Read the model definition and answer for the solid it produces. Units are mm, in the model's axes. A direction names the side the tool comes from. Round coordinates to 2 decimals unless told otherwise and drop trailing zeros. Order: outer loops, then holes, each group sorted by start corner. A loop starts at its lowest first (then second) coordinate and runs counter-clockwise, first axis right, second up. Notation, with made-up numbers: (30.5, 15) - (61.5, 15) arc R17 ccw to (61.5, 29) - close; hole circle Ø7 at (67, 80.25). An arc over 180 degrees is marked (long way). Answer as a JSON object with one key per item and string values. Group by question number.
Q1. Given pin 1 Ø5 at (x, y) = (292.43, 215.24) entering from -Z, flat-ended and moving along its own axis, determine where the tip first touches the part or whether it passes through.
Q2. Consider line 1 (Y direction, x = 303, z = 1.35); line 2 (Y direction, x = 310.5, z = 2.5); line 3 (Y direction, x = 301, z = 1.7). Determine where each line is inside the solid, lowest interval first.
Q3. A cutting plane is placed at A-A on x = 292.5. Determine the outline of the cut face in (y, z).
Q4. A tool of negligible diameter and unlimited length cuts with its end or side. For faces 1 (the flat face through (316.179, 224, 1)), 2 (the flat face through (251.929, 220, 1)), from which of +Z, -Z, +X, -X, +Y, -Y can it reach the whole face along a straight path? Write none if from no direction.
Q5. A cutting plane is placed at B-B on z = 0.5. Count the separate pieces of the cut face and the enclosed holes in it, and give its area (3 significant figures).
Q6. A cutting plane is placed at D-D on y = 212.25. Determine the outline of the cut face in (x, z), and give its area (3 significant figures).
Q7. A cutting plane is placed at C-C on y = 226.75. Determine the outline of the cut face in (x, z), and give its area (3 significant figures).
Q8. The mould has two halves that part along X. Classify faces 3 (the cylindrical face through (253.28, 212.03, 1.48)), 4 (the cylindrical face through (309.324, 216.256, 1.479)), 5 (the flat face through (350.929, 220, 1)): pulls with the +X half, pulls with the -X half, needs draft (parallel to the pull), parting line crosses it, or undercut.
```python
from build123d import *

# Parameters (mm, degrees)
MODEL_R                 = 1.5
SALIENTE_EXTRUIR1_DEPTH = 3


with BuildPart() as part:
    # Model → Saliente-Extruir1 (new body)
    with BuildSketch(Plane.XY):
        with BuildLine():
            Line((256.429131311, 228.742243614), (346.429131311, 228.742243614))
            ThreePointArc((346.429131311, 228.742243614), (349.611111826, 227.424224129), (350.929131311, 224.242243614))
            Line((350.929131311, 224.242243614), (350.929131311, 215.242243614))
            ThreePointArc((350.929131311, 215.242243614), (349.611111826, 212.060263099), (346.429131311, 210.742243614))
            Line((346.429131311, 210.742243614), (256.429131311, 210.742243614))
            ThreePointArc((256.429131311, 210.742243614), (253.247150795, 212.060263099), (251.929131311, 215.242243614))
            Line((251.929131311, 215.242243614), (251.929131311, 224.242243614))
            ThreePointArc((251.929131311, 224.242243614), (253.247150795, 227.424224129), (256.429131311, 228.742243614))
        make_face()
        with Locations((337.429131311, 215.242243614)):
            Circle(MODEL_R, mode=Mode.SUBTRACT)
        with Locations((319.429131311, 215.242243614)):
            Circle(MODEL_R, mode=Mode.SUBTRACT)
        with Locations((328.429131311, 215.242243614)):
            Circle(MODEL_R, mode=Mode.SUBTRACT)
        with Locations((310.429131311, 215.242243614)):
            Circle(MODEL_R, mode=Mode.SUBTRACT)
        with Locations((292.429131311, 215.242243614)):
            Circle(MODEL_R, mode=Mode.SUBTRACT)
        with Locations((301.429131311, 215.242243614)):
            Circle(MODEL_R, mode=Mode.SUBTRACT)
        with Locations((274.429131311, 215.242243614)):
            Circle(MODEL_R, mode=Mode.SUBTRACT)
        with Locations((283.429131311, 215.242243614)):
            Circle(MODEL_R, mode=Mode.SUBTRACT)
        with Locations((265.429131311, 215.242243614)):
            Circle(MODEL_R, mode=Mode.SUBTRACT)
        with Locations((256.429131311, 215.242243614)):
            Circle(MODEL_R, mode=Mode.SUBTRACT)
        with Locations((346.429131311, 215.242243614)):
            Circle(MODEL_R, mode=Mode.SUBTRACT)
        with BuildLine():
            Line((267.929131311, 222.617243614), (262.929131311, 222.617243614))
            ThreePointArc((262.929131311, 222.617243614), (262.398801225, 222.836913528), (262.179131311, 223.367243614))
            Line((262.179131311, 223.367243614), (262.179131311, 225.117243614))
            ThreePointArc((262.179131311, 225.117243614), (262.398801225, 225.6475737), (262.929131311, 225.867243614))
            Line((262.929131311, 225.867243614), (267.929131311, 225.867243614))
            ThreePointArc((267.929131311, 225.867243614), (268.459461397, 225.6475737), (268.679131311, 225.117243614))
            Line((268.679131311, 225.117243614), (268.679131311, 223.367243614))
            ThreePointArc((268.679131311, 223.367243614), (268.459461397, 222.836913528), (267.929131311, 222.617243614))
        make_face(mode=Mode.SUBTRACT)
        with BuildLine():
            Line((285.929131311, 222.617243614), (280.929131311, 222.617243614))
            ThreePointArc((280.929131311, 222.617243614), (280.398801225, 222.836913528), (280.179131311, 223.367243614))
            Line((280.179131311, 223.367243614), (280.179131311, 225.117243614))
            ThreePointArc((280.179131311, 225.117243614), (280.398801225, 225.6475737), (280.929131311, 225.867243614))
            Line((280.929131311, 225.867243614), (285.929131311, 225.867243614))
            ThreePointArc((285.929131311, 225.867243614), (286.459461397, 225.6475737), (286.679131311, 225.117243614))
            Line((286.679131311, 225.117243614), (286.679131311, 223.367243614))
            ThreePointArc((286.679131311, 223.367243614), (286.459461397, 222.836913528), (285.929131311, 222.617243614))
        make_face(mode=Mode.SUBTRACT)
        with BuildLine():
            Line((276.929131311, 222.617243614), (271.929131311, 222.617243614))
            ThreePointArc((271.929131311, 222.617243614), (271.398801225, 222.836913528), (271.179131311, 223.367243614))
            Line((271.179131311, 223.367243614), (271.179131311, 225.117243614))
            ThreePointArc((271.179131311, 225.117243614), (271.398801225, 225.6475737), (271.929131311, 225.867243614))
            Line((271.929131311, 225.867243614), (276.929131311, 225.867243614))
            ThreePointArc((276.929131311, 225.867243614), (277.459461397, 225.6475737), (277.679131311, 225.117243614))
            Line((277.679131311, 225.117243614), (277.679131311, 223.367243614))
            ThreePointArc((277.679131311, 223.367243614), (277.459461397, 222.836913528), (276.929131311, 222.617243614))
        make_face(mode=Mode.SUBTRACT)
        with BuildLine():
            Line((294.929131311, 222.617243614), (289.929131311, 222.617243614))
            ThreePointArc((289.929131311, 222.617243614), (289.398801225, 222.836913528), (289.179131311, 223.367243614))
            Line((289.179131311, 223.367243614), (289.179131311, 225.117243614))
            ThreePointArc((289.179131311, 225.117243614), (289.398801225, 225.6475737), (289.929131311, 225.867243614))
            Line((289.929131311, 225.867243614), (294.929131311, 225.867243614))
            ThreePointArc((294.929131311, 225.867243614), (295.459461397, 225.6475737), (295.679131311, 225.117243614))
            Line((295.679131311, 225.117243614), (295.679131311, 223.367243614))
            ThreePointArc((295.679131311, 223.367243614), (295.459461397, 222.836913528), (294.929131311, 222.617243614))
        make_face(mode=Mode.SUBTRACT)
        with BuildLine():
            Line((303.929131311, 222.617243614), (298.929131311, 222.617243614))
            ThreePointArc((298.929131311, 222.617243614), (298.398801225, 222.836913528), (298.179131311, 223.367243614))
            Line((298.179131311, 223.367243614), (298.179131311, 225.117243614))
            ThreePointArc((298.179131311, 225.117243614), (298.398801225, 225.6475737), (298.929131311, 225.867243614))
            Line((298.929131311, 225.867243614), (303.929131311, 225.867243614))
            ThreePointArc((303.929131311, 225.867243614), (304.459461397, 225.6475737), (304.679131311, 225.117243614))
            Line((304.679131311, 225.117243614), (304.679131311, 223.367243614))
            ThreePointArc((304.679131311, 223.367243614), (304.459461397, 222.836913528), (303.929131311, 222.617243614))
        make_face(mode=Mode.SUBTRACT)
        with BuildLine():
            Line((321.929131311, 222.617243614), (316.929131311, 222.617243614))
            ThreePointArc((316.929131311, 222.617243614), (316.398801225, 222.836913528), (316.179131311, 223.367243614))
            Line((316.179131311, 223.367243614), (316.179131311, 225.117243614))
            ThreePointArc((316.179131311, 225.117243614), (316.398801225, 225.6475737), (316.929131311, 225.867243614))
            Line((316.929131311, 225.867243614), (321.929131311, 225.867243614))
            ThreePointArc((321.929131311, 225.867243614), (322.459461397, 225.6475737), (322.679131311, 225.117243614))
            Line((322.679131311, 225.117243614), (322.679131311, 223.367243614))
            ThreePointArc((322.679131311, 223.367243614), (322.459461397, 222.836913528), (321.929131311, 222.617243614))
        make_face(mode=Mode.SUBTRACT)
        with BuildLine():
            Line((312.929131311, 222.617243614), (307.929131311, 222.617243614))
            ThreePointArc((307.929131311, 222.617243614), (307.398801225, 222.836913528), (307.179131311, 223.367243614))
            Line((307.179131311, 223.367243614), (307.179131311, 225.117243614))
            ThreePointArc((307.179131311, 225.117243614), (307.398801225, 225.6475737), (307.929131311, 225.867243614))
            Line((307.929131311, 225.867243614), (312.929131311, 225.867243614))
            ThreePointArc((312.929131311, 225.867243614), (313.459461397, 225.6475737), (313.679131311, 225.117243614))
            Line((313.679131311, 225.117243614), (313.679131311, 223.367243614))
            ThreePointArc((313.679131311, 223.367243614), (313.459461397, 222.836913528), (312.929131311, 222.617243614))
        make_face(mode=Mode.SUBTRACT)
        with BuildLine():
            Line((258.929131311, 222.617243614), (253.929131311, 222.617243614))
            ThreePointArc((253.929131311, 222.617243614), (253.398801225, 222.836913528), (253.179131311, 223.367243614))
            Line((253.179131311, 223.367243614), (253.179131311, 225.117243614))
            ThreePointArc((253.179131311, 225.117243614), (253.398801225, 225.6475737), (253.929131311, 225.867243614))
            Line((253.929131311, 225.867243614), (258.929131311, 225.867243614))
            ThreePointArc((258.929131311, 225.867243614), (259.459461397, 225.6475737), (259.679131311, 225.117243614))
            Line((259.679131311, 225.117243614), (259.679131311, 223.367243614))
            ThreePointArc((259.679131311, 223.367243614), (259.459461397, 222.836913528), (258.929131311, 222.617243614))
        make_face(mode=Mode.SUBTRACT)
        with BuildLine():
            Line((348.929131311, 222.617243614), (343.929131311, 222.617243614))
            ThreePointArc((343.929131311, 222.617243614), (343.398801225, 222.836913528), (343.179131311, 223.367243614))
            Line((343.179131311, 223.367243614), (343.179131311, 225.117243614))
            ThreePointArc((343.179131311, 225.117243614), (343.398801225, 225.6475737), (343.929131311, 225.867243614))
            Line((343.929131311, 225.867243614), (348.929131311, 225.867243614))
            ThreePointArc((348.929131311, 225.867243614), (349.459461397, 225.6475737), (349.679131311, 225.117243614))
            Line((349.679131311, 225.117243614), (349.679131311, 223.367243614))
            ThreePointArc((349.679131311, 223.367243614), (349.459461397, 222.836913528), (348.929131311, 222.617243614))
        make_face(mode=Mode.SUBTRACT)
        with BuildLine():
            Line((339.929131311, 222.617243614), (334.929131311, 222.617243614))
            ThreePointArc((334.929131311, 222.617243614), (334.398801225, 222.836913528), (334.179131311, 223.367243614))
            Line((334.179131311, 223.367243614), (334.179131311, 225.117243614))
            ThreePointArc((334.179131311, 225.117243614), (334.398801225, 225.6475737), (334.929131311, 225.867243614))
            Line((334.929131311, 225.867243614), (339.929131311, 225.867243614))
            ThreePointArc((339.929131311, 225.867243614), (340.459461397, 225.6475737), (340.679131311, 225.117243614))
            Line((340.679131311, 225.117243614), (340.679131311, 223.367243614))
            ThreePointArc((340.679131311, 223.367243614), (340.459461397, 222.836913528), (339.929131311, 222.617243614))
        make_face(mode=Mode.SUBTRACT)
        with BuildLine():
            Line((330.929131311, 222.617243614), (325.929131311, 222.617243614))
            ThreePointArc((325.929131311, 222.617243614), (325.398801225, 222.836913528), (325.179131311, 223.367243614))
            Line((325.179131311, 223.367243614), (325.179131311, 225.117243614))
            ThreePointArc((325.179131311, 225.117243614), (325.398801225, 225.6475737), (325.929131311, 225.867243614))
            Line((325.929131311, 225.867243614), (330.929131311, 225.867243614))
            ThreePointArc((330.929131311, 225.867243614), (331.459461397, 225.6475737), (331.679131311, 225.117243614))
            Line((331.679131311, 225.117243614), (331.679131311, 223.367243614))
            ThreePointArc((331.679131311, 223.367243614), (331.459461397, 222.836913528), (330.929131311, 222.617243614))
        make_face(mode=Mode.SUBTRACT)
    extrude(amount=SALIENTE_EXTRUIR1_DEPTH)


solid = part.part
```
Result set:
{
 "1": {"pin 1": "stops at z = 0"},
 "2": {"line 1": "y = 210.74 to 222.62, 225.87 to 228.74", "line 2": "y = 210.74 to 213.74, 216.74 to 222.62, 225.87 to 228.74", "line 3": "y = 210.74 to 213.8, 216.68 to 222.62, 225.87 to 228.74"},
 "3": {"outline": "(210.74, 0) - (213.74, 0) - (213.74, 3) - (210.74, 3) - close; (216.74, 0) - (222.62, 0) - (222.62, 3) - (216.74, 3) - close; (225.87, 0) - (228.74, 0) - (228.74, 3) - (225.87, 3) - close"},
 "4": {"face 1": "+Z, -Z", "face 2": "+Z, -Z, -X, +Y, -Y"},
 "5": {"separate pieces": "1", "enclosed holes": "22", "area": "1,460 mm²"},
 "6": {"outline": "(253.07, 0) - (349.79, 0) - (349.79, 3) - (253.07, 3) - close", "area": "290 mm²"},
 "7": {"outline": "(252.69, 0) - (350.17, 0) - (350.17, 3) - (252.69, 3) - close", "area": "292 mm²"},
 "8": {"face 3": "pulls with the -X half", "face 4": "undercut", "face 5": "pulls with the +X half"}
}
